For this review, take the finished solid that the model builds, in its own axes (mm). Give positions to 0.01 mm unless a question says otherwise; leave off trailing zeros. Loops run counter-clockwise (first coordinate to the right, second up) from the corner with the lowest first, then second, coordinate; pieces in that order, holes last. Notation, with made-up numbers: (13.25, 19) - (24.25, 19) arc R19 cw to (24.25, 25) - close; hole circle Ø2 at (1, -29). An arc over 180 degrees is marked (long way). Put each result on its own line as item: value.
from build123d import *

# Parameters (mm, degrees)
F1_DEPTH = 2.38125
F2_R     = 2.38125
F3_DEPTH = 25.4
F5_DEPTH = 25.4


with BuildPart() as f1:
    # F0 (on Front) → F1 (new body)
    with BuildSketch(Plane.XZ):
        with BuildLine():
            Line((60.325, 19.05), (7.9375, 19.05))
            ThreePointArc((7.9375, 19.05), (2.32484, 16.72516), (0, 11.1125))
            Line((0, 11.1125), (0, 0))
            Line((0, 0), (9.525, 0))
            Line((9.525, 0), (12.110345, 7.626242))
            ThreePointArc((12.110345, 7.626242), (13.602572, 9.611517), (15.981838, 10.323664))
            Line((15.981838, 10.323664), (60.325, 12.7))
            Line((60.325, 12.7), (60.325, 19.05))
        make_face()
    extrude(amount=F1_DEPTH)

    # F2 (on face) → F3 (cut)
    with BuildSketch(Plane.XZ.offset(2.38125)):
        with Locations((7.9375, 11.1125)):
            Circle(F2_R)
    extrude(amount=-F3_DEPTH, mode=Mode.SUBTRACT)

    # F4 (on face) → F5 (cut)
    with BuildSketch(Plane.XY.offset(19.05)):
        Polygon((60.325, 0), (48.834524, 0), (60.325, -0.79375), align=None)
        Polygon((60.325, -2.38125), (60.325, -1.5875), (48.834524, -2.38125), align=None)
    extrude(amount=-F5_DEPTH, mode=Mode.SUBTRACT)


solid = f1.part
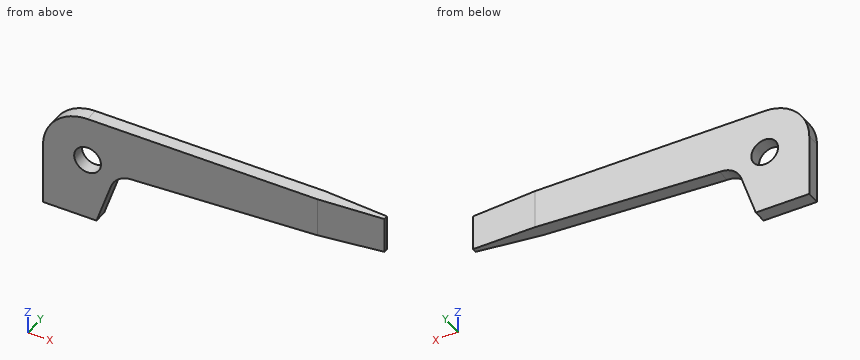
1) Wall thickness on line 1 (Z direction, x = 49, y = -2.3); line 2 (Z direction, x = 28.5, y = -0.3); line 3 (X direction, y = -2.1, z = 8.25): over which ranges is each line inside the solid? List them lowest first.
Geometry check:
line 1: z = 12.09 to 19.05
line 2: z = 10.99 to 19.05
line 3: x = 0 to 12.38
2) Insertion check: pin 1 Ø5.5 at (x, z) = (7.94, 11.11) entering from +Y; pin 2 Ø1 at (y, z) = (-0.5, 14.5) entering from -X. Each pin has a flat end and moves straight along its axis. Give the tip position at first contact, or say it passes through.
Geometry check:
pin 1: stops at y = 0
pin 2: stops at x = 0.54
3) Take a section at B-B on x = 18. State the section outline as (y, z) points.
Geometry check:
outline: (-2.38, 10.43) - (0, 10.43) - (0, 19.05) - (-2.38, 19.05) - close
4) Take a section at A-A on z = 5. State the section outline as (x, y) points, and give its area (3 significant figures).
Geometry check:
outline: (0, -2.38) - (11.22, -2.38) - (11.22, 0) - (0, 0) - close
area: 26.7 mm²
